Solid Edge part; units mm, degrees
sketch "Sketch1" plane through (0, 0, 0) normal (-0.0523, 0, 0.9986) x (0, 1, 0)
  line L0 (1.125, -1) -> (1.125, 1)
  line L1 (1.125, 1) -> (-1.125, 1)
  line L2 (-1.125, 1) -> (-1.125, -1)
  line L3 (-1.125, -1) -> (1.125, -1)
extrude "ExtrudedProtrusion_1" add sketch "Sketch1" along normal blind 48.12
sketch "Sketch2" plane through (-0.2574, 0, 24.0194) normal (0.9986, 0, 0.0523) x (0.0523, 0, -0.9986)
  line L0 (24, -1.125) -> (24, 1.125)
  line L1 (23.8821, 1.125) -> (24, 1.125)
  line L2 (24, -1.125) -> (23.8821, 1.125)
extrude "Cutout1" cut sketch "Sketch2" against normal up to vertex (2 mm away)
properties material "Stainless Steel, 420"
Read the model definition and answer for the solid it produces. Units are mm, in the model's axes. Coordinates: 2 decimals unless noted, no trailing zeros. Loops run counter-clockwise (first coordinate to the right, second up) from the corner with the lowest first, then second, coordinate; pieces in that order, holes last. Notation, with made-up numbers: (80.25, 32.5) -> (118.25, 32.5) arc R25 ccw to (118.25, 56.5) -> close; hole circle Ø7 at (18.5, 41). An arc over 180 degrees is marked (long way). Return JSON: item names as keys, results as strings.
Item 1: Find section C-C (z = 27). Determine the outline of the cut face in (x, y) (3 decimals), plus the area to 3 significant figures.
Answers:
{"outline": "(-2.416, -1.125) -> (-0.414, -1.125) -> (-0.414, 1.125) -> (-2.416, 1.125) -> close", "area": "4.51 mm2"}
Item 2: A flat-ended cylindrical pin translates along its axis: P1, Ø1, axis at y = 0, z = 42, coming from the -X side. Find the tip coordinate at first contact, or state that the pin passes through.
Answers:
{"P1": "stops at x = -3.23"}
Item 3: For a pull along Y with two mould halves and no side action, classify faces 1 (the flat face through (-2.532, 0.016, 48.053)), 2 (the flat face through (-1, 1.125, 24)), 3 (the flat face through (-1, -1.125, 24)) as +Y half, -Y half, draft (parallel to the pull), parting line (faces both ways), or undercut.
Answers:
{"face 1": "draft", "face 2": "+Y half", "face 3": "-Y half"}
Item 4: Find the intervals of material crossed by probe 1 along X at (y, z) = (-0.4, 30.5); probe 2 along X at (y, z) = (0.35, 16), in increasing order.
Answers:
{"probe 1": "x = -2.6 to -0.6", "probe 2": "x = -1.84 to 0.16"}
Item 5: Find section A-A (y = -0.5). Determine the outline of the cut face in (x, z) (3 decimals), plus the area to 3 significant figures.
Answers:
{"outline": "(-3.517, 48.002) -> (-1, -0.02) -> (0.997, 0.085) -> (-1.52, 48.106) -> close", "area": "96.2 mm2"}
